```python
from build123d import *

# Parameters (mm, degrees)
F1_DEPTH = 25
F2_R     = 11
F3_R     = 3
F4_R     = 3
F6_D     = 10.5
F8_D     = 10.5


with BuildPart() as f1:
    # F0 (on Top) → F1 (new body)
    with BuildSketch(Plane.XY):
        with BuildLine():
            ThreePointArc((-42.475013, 13.076226), (-42.211382, 17.110535), (-41.424972, 21.076226))
            Line((-41.424972, 21.076226), (-66.424972, 21.076226))
            Line((-66.424972, 21.076226), (-66.424972, 13.076226))
            Line((-66.424972, 13.076226), (-42.475013, 13.076226))
        make_face()
        with BuildLine():
            Line((43.474945, 21.076226), (18.474945, 21.076226))
            ThreePointArc((18.474945, 21.076226), (19.261355, 17.110535), (19.524987, 13.076226))
            Line((19.524987, 13.076226), (43.474945, 13.076226))
            Line((43.474945, 13.076226), (43.474945, 21.076226))
        make_face()
        with BuildLine():
            ThreePointArc((-3.475013, 43.026184), (-7.440705, 43.812595), (-11.475013, 44.076226))
            ThreePointArc((-11.475013, 44.076226), (-15.509322, 43.812595), (-19.475013, 43.026184))
            ThreePointArc((-19.475013, 43.026184), (-33.395323, 34.996536), (-41.424972, 21.076226))
            ThreePointArc((-41.424972, 21.076226), (-42.211382, 17.110535), (-42.475013, 13.076226))
            Line((-42.475013, 13.076226), (-35.475013, 13.076226))
            ThreePointArc((-35.475013, 13.076226), (-28.445576, 30.046789), (-11.475013, 37.076226))
            ThreePointArc((-11.475013, 37.076226), (5.495549, 30.046789), (12.524987, 13.076226))
            Line((12.524987, 13.076226), (19.524987, 13.076226))
            ThreePointArc((19.524987, 13.076226), (19.261355, 17.110535), (18.474945, 21.076226))
            ThreePointArc((18.474945, 21.076226), (10.445297, 34.996536), (-3.475013, 43.026184))
        make_face()
        with BuildLine():
            ThreePointArc((-19.475013, 43.026184), (-15.509322, 43.812595), (-11.475013, 44.076226))
            ThreePointArc((-11.475013, 44.076226), (-7.440705, 43.812595), (-3.475013, 43.026184))
            Line((-3.475013, 43.026184), (-3.475013, 68.026184))
            Line((-3.475013, 68.026184), (-19.475013, 68.026184))
            Line((-19.475013, 68.026184), (-19.475013, 43.026184))
        make_face()
    extrude(amount=F1_DEPTH)

    # F2
    f2_edges = [f1.edges().sort_by_distance(p)[0] for p in [
        (43.474945, 17.076226, 0),
        (43.474945, 17.076226, 25),
        (-66.424972, 17.076226, 25),
        (-66.424972, 17.076226, 0),
        (-11.475013, 68.026184, 0),
        (-11.475013, 68.026184, 25),
    ]]
    fillet(f2_edges, radius=F2_R)

    # F3
    f3_edges = [f1.edges().sort_by_distance(p)[0] for p in [
        (-35.475013, 13.076226, 12.5),
        (12.524987, 13.076226, 12.5),
    ]]
    fillet(f3_edges, radius=F3_R)

    # F4
    f4_edges = [f1.edges().sort_by_distance(p)[0] for p in [
        (-41.424972, 21.076226, 12.5),
        (18.474945, 21.076226, 12.5),
        (-3.475013, 43.026184, 12.5),
        (-19.475013, 43.026184, 12.5),
    ]]
    fillet(f4_edges, radius=F4_R)

    # F6 (through all)
    with Locations(Plane(origin=(0, 21.076226, 0), x_dir=(-1, 0, 0), z_dir=(0, 1, 0))):
        with Locations((55.174972, 12.5), (-32.224945, 12.5)):
            Hole(F6_D / 2)

    # F8 (through all)
    with Locations(Plane.YZ.offset(-3.475013)):
        with Locations((56.776184, 12.5)):
            Hole(F8_D / 2)


solid = f1.part
```
The model under review builds one solid part; all positions refer to its coordinate system, in mm. A direction names the side the tool comes from. Round coordinates to 2 decimals unless told otherwise and drop trailing zeros. Order: outer loops, then holes, each group sorted by start corner. A loop starts at its lowest first (then second) coordinate and runs counter-clockwise, first axis right, second up. Notation, with made-up numbers: (32, 44) -> (43, 44) arc R22 ccw to (43, 67) -> close; hole circle Ø2 at (70, 40.25). An arc over 180 degrees is marked (long way). Use a Markdown table: item, result.
Q1. We need section C-C on x = -51.5. Write out the cut boundary in (y, z).
Values:
| item | result |
|---|---|
| outline | (13.08, 0) -> (21.08, 0) -> (21.08, 8.75) -> (13.08, 8.75) -> close; (13.08, 16.25) -> (21.08, 16.25) -> (21.08, 25) -> (13.08, 25) -> close |
Q2. Mouldability with a two-part tool opening along X and no side actions: class faces 1 (the cylindrical face through (-41.923, 21.621, 12.675)), 2 (the cylindrical face through (-50.17, 17.02, 14.08)), 3 (the cylindrical face through (-11.59, 64.89, 21.69)) as +X half, -X half, draft (parallel to the pull), parting line (faces both ways), or undercut.
Values:
| item | result |
|---|---|
| face 1 | -X half |
| face 2 | undercut |
| face 3 | draft |
Q3. For line 1 (X direction, y = 27.5, z = 16.25) (3 decimals); line 2 (Y direction, x = -12, z = 9.5); line 3 (X direction, y = 27, z = 5.25), list the stretches that pass through material, from the lowest coordinate up.
Values:
| item | result |
|---|---|
| line 1 | x = -38.915 to -30.657, 7.707 to 15.965 |
| line 2 | y = 37.07 to 52.47, 61.08 to 67.92 |
| line 3 | x = -39.17 to -31.02, 8.07 to 16.22 |
Q4. We need section D-D on y = 17.5. Write out the cut boundary in (x, z), then the cut area to 3 significant figures.
Values:
| item | result |
|---|---|
| outline | (-66.42, 11) arc R11 ccw to (-55.42, 0) -> (-35.06, 0) -> (-35.06, 25) -> (-55.42, 25) arc R11 ccw to (-66.42, 14) -> close; (12.11, 0) -> (32.47, 0) arc R11 ccw to (43.47, 11) -> (43.47, 14) arc R11 ccw to (32.47, 25) -> (12.11, 25) -> close; hole circle Ø10.5 at (-55.17, 12.5); hole circle Ø10.5 at (32.22, 12.5) |
| area | 1,290 mm^2 |
Q5. Tool access review of faces 4 (the cylindrical face through (-36.33, 13.82, 12.68)), 5 (the cylindrical face through (-63.29, 17.02, 3.31)), 6 (the flat face through (-50, 21.076, 10)), 7 (the flat face through (-3.475, 51, 12)), 8 (the cylindrical face through (28.355, 17.02, 16.048)): name each direction out of +Z, -Z, +X, -X, +Y, -Y from which nothing blocks a thin tool from reaching the whole face with its end or side.
Values:
| item | result |
|---|---|
| face 4 | +Z, -Z, -Y |
| face 5 | -Z, -X, +Y, -Y |
| face 6 | +Z, -Z, -X, +Y |
| face 7 | +Z, -Z, +X, +Y |
| face 8 | +Y, -Y |
Q6. Clearance check with flat-ended pins moving along their axes: P1, Ø10, axis at x = -6, y = 57.5, coming from the -Z side; P2, Ø2, axis at x = -52, z = 3.5, coming from the +Y side; P3, Ø13.5, axis at y = 56.78, z = 12.5, coming from the -X side (3 decimals). State where each tip first meets the part, or that it passes through.
Values:
| item | result |
|---|---|
| P1 | stops at z = 0 |
| P2 | stops at y = 21.08 |
| P3 | stops at x = -19.475 |
Q7. We need section A-A on z = 12.5. State how many separate pieces and enclosed holes the cut face has, then the cut area to 3 significant figures.
Values:
| item | result |
|---|---|
| separate pieces | 4 |
| enclosed holes | 0 |
| area | 1,050 mm^2 |
Q8. We need section B-B on y = 55.5. Write out the cut boundary in (x, z).
Values:
| item | result |
|---|---|
| outline | (-19.48, 0) -> (-3.48, 0) -> (-3.48, 7.41) -> (-19.48, 7.41) -> close; (-19.48, 17.59) -> (-3.48, 17.59) -> (-3.48, 25) -> (-19.48, 25) -> close |
